from build123d import *
from build123d.topology import SkipClean

# Parameters (mm, degrees)
SKETCH1_W           = 41.99999943
SKETCH1_H           = 32.99999982
BOSS_EXTRUDE1_DEPTH = 2
FILLET1_R           = 4
SKETCH3_R           = 1.65
CUT_EXTRUDE1_DEPTH  = 2
SKETCH5_W           = 41.99999943
SKETCH5_H           = 16
BOSS_EXTRUDE3_DEPTH = 2
SKETCH6_R           = 1.65
SKETCH6_R_2         = 1.656480043
CUT_EXTRUDE2_DEPTH  = 2
FILLET2_R           = 17
FILLET3_R           = 4
SKETCH7_W           = 9
SKETCH7_H           = 44.079753615
BOSS_EXTRUDE4_DEPTH = 2
CUT_EXTRUDE3_DEPTH  = 2
FILLET4_R           = 4
SKETCH9_R           = 1
BOSS_EXTRUDE5_DEPTH = 10
SKETCH10_W          = 1.2
SKETCH10_H          = 2
BOSS_EXTRUDE6_DEPTH = 2
SKETCH11_W          = 4.5
SKETCH11_H          = 2
BOSS_EXTRUDE7_DEPTH = 12
CUT_EXTRUDE4_DEPTH  = 10
SKETCH13_W          = 2
SKETCH13_H          = 4.75
CUT_EXTRUDE5_DEPTH  = 2
BOSS_EXTRUDE8_START = 2
SKETCH15_W          = 4.5
SKETCH15_H          = 12
SKETCH15_R          = 1.05
BOSS_EXTRUDE8_DEPTH = 2


with BuildPart() as part:
    # Sketch1 → Boss-Extrude1 (new body)
    with BuildSketch(Plane(origin=(0, 0, 0), x_dir=(1, 0, 0), z_dir=(0, 1, 0))):
        with Locations((20.999999715, 16.49999991)):
            Rectangle(SKETCH1_W, SKETCH1_H)
    extrude(amount=BOSS_EXTRUDE1_DEPTH)

    # Fillet1
    fillet1_edges = [part.edges().sort_by_distance(p)[0] for p in [
        (0, 1, -32.99999982),
        (41.99999943, 1, -32.99999982),
        (41.99999943, 1, 0),
        (0, 1, 0),
    ]]
    fillet(fillet1_edges, radius=FILLET1_R)

    # Sketch3 → Cut-Extrude1 (cut)
    with BuildSketch(Plane.XZ):
        with Locations(Location((3.75, -3.5, 0), (0, 0, 270))):
            Circle(SKETCH3_R)
        with Locations(Location((3.75, -29.499999821, 0), (0, 0, 270))):
            Circle(SKETCH3_R)
        with Locations(Location((38.249999434, -28.499999821, 0), (0, 0, 270))):
            Circle(SKETCH3_R)
        with Locations(Location((38.249999434, -4.5, 0), (0, 0, 270))):
            Circle(SKETCH3_R)
    extrude(amount=-CUT_EXTRUDE1_DEPTH, mode=Mode.SUBTRACT)

    # Sketch5 → Boss-Extrude3 (add)
    with BuildSketch(Plane.XZ):
        with Locations((20.999999715, -36.079753615)):
            Rectangle(SKETCH5_W, SKETCH5_H)
    extrude(amount=-BOSS_EXTRUDE3_DEPTH)

    # Sketch6 → Cut-Extrude2 (cut)
    with BuildSketch(Plane.XZ):
        with Locations(Location((38.249999434, -28.499999821, 0), (0, 0, 270))):
            Circle(SKETCH6_R)
        with Locations(Location((3.747696905, -29.506056777, 0), (0, 0, 270))):
            Circle(SKETCH6_R_2)
    extrude(amount=-CUT_EXTRUDE2_DEPTH, mode=Mode.SUBTRACT)

    # Fillet2
    fillet2_edges = [part.edges().sort_by_distance(p)[0] for p in [
        (41.99999943, 1, -44.079753615),
    ]]
    fillet(fillet2_edges, radius=FILLET2_R)

    # Fillet3
    fillet3_edges = [part.edges().sort_by_distance(p)[0] for p in [
        (0, 1, -44.079753615),
    ]]
    fillet(fillet3_edges, radius=FILLET3_R)

    # Sketch7 → Boss-Extrude4 (add)
    with BuildSketch(Plane.XZ):
        with Locations((-0.5, -22.039876808)):
            Rectangle(SKETCH7_W, SKETCH7_H)
    extrude(amount=-BOSS_EXTRUDE4_DEPTH)

    # Sketch8 → Cut-Extrude3 (cut)
    with SkipClean():  # the faces are left unmerged after this step: merging them gives an invalid solid
        with BuildSketch(Plane.XZ):
            with BuildLine():
                ThreePointArc((4, -5.130950643), (5.001998403, -4.574709263), (5.4, -3.5))
                ThreePointArc((5.4, -3.5), (5.001998403, -2.425290737), (4, -1.869049357))
                Line((4, -1.869049357), (4, -5.130950643))
            make_face()
            with BuildLine():
                Line((4, -5.130950643), (4, -1.869049357))
                ThreePointArc((4, -1.869049357), (2.1, -3.5), (4, -5.130950643))
            make_face()
            with BuildLine():
                ThreePointArc((4, -1.869049357), (5.4, -3.5), (4, -5.130950643))
                Line((4, -5.130950643), (4, -1.869049357))
            make_face()
            with BuildLine():
                ThreePointArc((4, -27.86890398), (5.404176948, -29.506056777), (4, -31.143209574))
                Line((4, -31.143209574), (4, -27.86890398))
            make_face()
            with BuildLine():
                ThreePointArc((5.404176948, -29.506056777), (5.402815419, -29.43890888), (5.398733067, -29.371871366))
                ThreePointArc((5.398733067, -29.371871366), (4.96029858, -28.377551876), (4, -27.86890398))
                Line((4, -27.86890398), (4, -31.143209574))
                ThreePointArc((4, -31.143209574), (5.005047527, -30.584479489), (5.404176948, -29.506056777))
            make_face()
            with BuildLine():
                Line((4, -31.143209574), (4, -27.86890398))
                ThreePointArc((4, -27.86890398), (2.091216862, -29.506056777), (4, -31.143209574))
            make_face()
        extrude(amount=-CUT_EXTRUDE3_DEPTH, mode=Mode.SUBTRACT)

    # Fillet4
    fillet4_edges = [part.edges().sort_by_distance(p)[0] for p in [
        (-5, 1, -44.079753615),
        (-5, 1, 0),
    ]]
    fillet(fillet4_edges, radius=FILLET4_R)

    # Sketch9 → Boss-Extrude5 (add)
    with BuildSketch(Plane.XZ):
        with BuildLine():
            Line((19.99999943, -38.62499991), (19.99999943, -28.49999991))
            Line((19.99999943, -28.49999991), (6.573975303, -28.49999991))
            ThreePointArc((6.573975303, -28.49999991), (6.703947503, -28.995584051), (6.747696905, -29.506056777))
            ThreePointArc((6.747696905, -29.506056777), (4.543595006, -32.398555042), (1.16999943, -31.040812694))
            Line((1.16999943, -31.040812694), (1.16999943, -43.74999991))
            Line((1.16999943, -43.74999991), (19.99999943, -43.74999991))
            Line((19.99999943, -43.74999991), (19.99999943, -38.62499991))
        make_face()
        with Locations(Location((17.99999943, -41.74999991, 0), (0, 0, 270))):
            Circle(SKETCH9_R, mode=Mode.SUBTRACT)
        with Locations(Location((17.99999943, -30.49999991, 0), (0, 0, 270))):
            Circle(SKETCH9_R, mode=Mode.SUBTRACT)
    extrude(amount=BOSS_EXTRUDE5_DEPTH)

    # Sketch10 → Boss-Extrude6 (add)
    with BuildSketch(Plane(origin=(0, 2, 0), x_dir=(1, 0, 0), z_dir=(0, 1, 0))):
        with Locations((42.59999943, 13.15)):
            Rectangle(SKETCH10_W, SKETCH10_H)
    extrude(amount=-BOSS_EXTRUDE6_DEPTH)

    # Sketch11 → Boss-Extrude7 (add)
    with BuildSketch(Plane.XZ):
        with Locations((40.94999943, -13.15)):
            Rectangle(SKETCH11_W, SKETCH11_H)
        with Locations((12.894917885, -13.15)):
            Rectangle(SKETCH11_W, SKETCH11_H)
    extrude(amount=BOSS_EXTRUDE7_DEPTH)

    # Sketch12 → Cut-Extrude4 (cut)
    with BuildSketch(Plane.XY.offset(-12.15)):
        with BuildLine():
            ThreePointArc((41.694917885, -6), (41.66275253, -5.742099563), (41.568227151, -5.5))
            ThreePointArc((41.568227151, -5.5), (39.594917885, -6), (41.568227151, -6.5))
            ThreePointArc((41.568227151, -6.5), (41.66275253, -6.257900437), (41.694917885, -6))
        make_face()
        with BuildLine():
            ThreePointArc((12.221608619, -5.5), (12.094917885, -6), (12.221608619, -6.5))
            ThreePointArc((12.221608619, -6.5), (13.402818322, -7.017834645), (14.194917885, -6))
            ThreePointArc((14.194917885, -6), (13.402818322, -4.982165355), (12.221608619, -5.5))
        make_face()
    extrude(amount=-CUT_EXTRUDE4_DEPTH, mode=Mode.SUBTRACT)

    # Sketch13 → Cut-Extrude5 (cut)
    with BuildSketch(Plane(origin=(19.99999943, 0, 0), x_dir=(0, 0, -1), z_dir=(1, 0, 0))):
        with Locations((29.49999991, -6.125)):
            Rectangle(SKETCH13_W, SKETCH13_H)
    extrude(amount=-CUT_EXTRUDE5_DEPTH, mode=Mode.SUBTRACT)

    # Sketch15 → Boss-Extrude8 (add)
    # profile 1 of 2: a face of its own
    with BuildSketch(Plane.XY.offset(-12.15).offset(BOSS_EXTRUDE8_START)):
        with Locations((12.894917885, -6)):
            Rectangle(SKETCH15_W, SKETCH15_H)
        with Locations((13.144917885, -6)):
            Circle(SKETCH15_R, mode=Mode.SUBTRACT)
    # profile 2 of 2: a face of its own
    with BuildSketch(Plane.XY.offset(-12.15).offset(BOSS_EXTRUDE8_START)):
        Polygon((41.99999943, 2), (41.99999943, 0), (38.69999943, 0), (38.69999943, -12), (43.19999943, -12), (43.19999943, 2), align=None)
        with Locations((40.644917885, -6)):
            Circle(SKETCH15_R, mode=Mode.SUBTRACT)
    extrude(amount=-BOSS_EXTRUDE8_DEPTH)


solid = part.part
Verification items for the finished model (mm, model axes). A direction names the side the tool comes from. Give positions to 0.01 mm unless a question says otherwise; leave off trailing zeros. Loops run counter-clockwise (first coordinate to the right, second up) from the corner with the lowest first, then second, coordinate; pieces in that order, holes last.
1. Go/stop test with flat-tipped pins: P1, Ø4, axis at x = 38.25, z = -28.5, coming from the -Y side; P2, Ø13, axis at x = 20, z = -18, coming from the -Y side; P3, Ø5, axis at x = 14.5, y = -3, coming from the -Z side; P4, Ø2, axis at x = 18.5, z = -42, coming from the -Y side. Record where each tip stops, or that it passes through.
Derived:
P1: stops at y = 0
P2: stops at y = -12
P3: stops at z = -43.75
P4: stops at y = -10
2. Cross-section at B-B on x = 40.5. Record the cut outline in (y, z), and give its area (3 significant figures).
Derived:
outline: (-12, -14.15) - (-7.04, -14.15) - (-7.04, -10.15) - (-12, -10.15) - close; (-4.96, -14.15) - (0, -14.15) - (0, -34.06) - (2, -34.06) - (2, -0.88) - (0, -0.88) - (0, -10.15) - (-4.96, -10.15) - close
area: 106 mm2
3. Cross-section at C-C on z = -34.5. Record the cut outline in (x, y), and give its area (3 significant figures).
Derived:
outline: (-5, 0) - (1.17, 0) - (1.17, -10) - (20, -10) - (20, 0) - (40.3, 0) - (40.3, 2) - (-5, 2) - close
area: 279 mm2
4. Cross-section at A-A on y = -2. Record the cut outline in (x, z).
Derived:
outline: (1.17, -43.75) - (20, -43.75) - (20, -28.5) - (6.57, -28.5) arc R3 cw to (1.17, -31.04) - close; (10.64, -14.15) - (15.14, -14.15) - (15.14, -10.15) - (10.64, -10.15) - close; (38.7, -14.15) - (43.2, -14.15) - (43.2, -10.15) - (38.7, -10.15) - close; hole circle Ø2 at (18, -41.75); hole circle Ø2 at (18, -30.5)
5. Cross-section at D-D on x = 0. Record the cut outline in (y, z), and give its area (3 significant figures).
Derived:
outline: (0, -44.08) - (2, -44.08) - (2, 0) - (0, 0) - close
area: 88.2 mm2
6. Release check for a two-part mould opening along Y. For faces 5 (the flat face through (41.4, -4.9, -14.15)), 6 (the cylindrical face through (13.506, -6.986, -12.566)), 7 (the flat face through (10, -10, -36)) record: +Y half, -Y half, draft (parallel to the pull), parting line (faces both ways), or undercut.
Derived:
face 5: draft
face 6: undercut
face 7: -Y half
7. Material ranges on probe 1 along X at (y, z) = (-6, -10.6); probe 2 along X at (y, z) = (-6.25, -32); probe 3 along X at (y, z) = (0.9, -28.5), recorded low to high.
Derived:
probe 1: x = 10.64 to 12.09, 14.19 to 15.14, 38.7 to 39.59, 41.69 to 43.2
probe 2: x = 1.17 to 2.08, 5.42 to 20
probe 3: x = -5 to 2.43, 5.06 to 36.6, 39.9 to 41.94
8. Tool access check on faces 1 (the flat face through (18, 0, -42)), 2 (the flat face through (1.17, -5, -37)), 3 (the flat face through (20, -5, -36)), 4 (the flat face through (11.9, -5.9, -14.15)). Record the directions out of +Z, -Z, +X, -X, +Y, -Y that give a thin tool (end or side, any length) a straight path to the whole face; none if there is none.
Derived:
face 1: -Y
face 2: +Z, -Z, -X, -Y
face 3: +Z, -Z, +X, -Y
face 4: +X, -X, -Y
